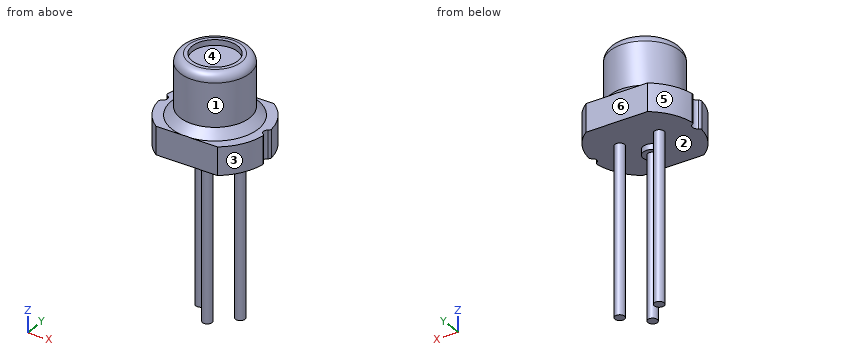
```python
from build123d import *

# Parameters (mm, degrees)
BOSS_EXTRUDE1_DEPTH = 1
SKETCH3_R           = 1.25
BOSS_EXTRUDE2_DEPTH = 2.15
CHAMFER1_SIZE       = 0.3
FILLET1_R           = 0.3
SKETCH4_R           = 0.817963918
CUT_EXTRUDE1_DEPTH  = 0.2
SKETCH5_R           = 0.175
BOSS_EXTRUDE3_DEPTH = 6
SKETCH6_R           = 0.340201154
BOSS_EXTRUDE4_DEPTH = 0.2


with BuildPart() as part:
    # Sketch1 → Boss-Extrude1 (new body)
    with BuildSketch(Plane.XY):
        with BuildLine():
            Line((-1.112834219, 1.54), (1.112834219, 1.54))
            ThreePointArc((1.112834219, 1.54), (1.63498089, 0.967903657), (1.885416667, 0.2349553))
            ThreePointArc((1.885416667, 0.2349553), (1.874554764, 0.175784903), (1.831710526, 0.133553539))
            ThreePointArc((1.831710526, 0.133553539), (1.75, 0), (1.831710526, -0.133553539))
            ThreePointArc((1.831710526, -0.133553539), (1.874554764, -0.175784903), (1.885416667, -0.2349553))
            ThreePointArc((1.885416667, -0.2349553), (1.63498089, -0.967903657), (1.112834219, -1.54))
            Line((1.112834219, -1.54), (-1.112834219, -1.54))
            ThreePointArc((-1.112834219, -1.54), (-1.626419084, -0.982222462), (-1.881, -0.268027984))
            ThreePointArc((-1.881, -0.268027984), (-1.869896042, -0.206231776), (-1.824142857, -0.163235088))
            ThreePointArc((-1.824142857, -0.163235088), (-1.72, 0), (-1.824142857, 0.163235088))
            ThreePointArc((-1.824142857, 0.163235088), (-1.869896042, 0.206231776), (-1.881, 0.268027984))
            ThreePointArc((-1.881, 0.268027984), (-1.626419084, 0.982222462), (-1.112834219, 1.54))
        make_face()
    extrude(amount=BOSS_EXTRUDE1_DEPTH)

    # Sketch3 → Boss-Extrude2 (add)
    with BuildSketch(Plane.XY.offset(1)):
        with Locations(Location((0, 0, 0), (0, 0, 180))):
            Circle(SKETCH3_R)
    extrude(amount=BOSS_EXTRUDE2_DEPTH)

    # Chamfer1
    # the kernel refuses this chamfer: 0.3 mm, written as the material it adds along each edge
    with BuildSketch(Plane(origin=(0, 0, 1), x_dir=(-1, 0, 0), z_dir=(0, 1, 0))) as chamfer1_piece_1_section:
        Polygon((1.25 + CHAMFER1_SIZE, 0), (1.25, CHAMFER1_SIZE), (1.25, 0), align=None)
    chamfer1_piece_1 = revolve(axis=Axis((0, 0, 1), (0, 0, 1)), mode=Mode.PRIVATE)
    chamfer1_piece_1 = split(chamfer1_piece_1, bisect_by=Plane(origin=(1.394706395, -1.54, 1.144706395), z_dir=(0, 1, 0)), keep=Keep.TOP, mode=Mode.PRIVATE)
    chamfer1_piece_1 = split(chamfer1_piece_1, bisect_by=Plane(origin=(1.394706395, 1.54, 1.144706395), z_dir=(0, -1, 0)), keep=Keep.TOP, mode=Mode.PRIVATE)
    add(chamfer1_piece_1)

    # Fillet1
    fillet1_edges = [part.edges().sort_by_distance(p)[0] for p in [
        (1.25, 0, 3.15),
    ]]
    fillet(fillet1_edges, radius=FILLET1_R)

    # Sketch4 → Cut-Extrude1 (cut)
    with BuildSketch(Plane.XY.offset(3.15)):
        Circle(SKETCH4_R)
    extrude(amount=-CUT_EXTRUDE1_DEPTH, mode=Mode.SUBTRACT)

    # Sketch5 → Boss-Extrude3 (add)
    with BuildSketch(Plane.XY):
        with Locations((0.715, 0.3)):
            Circle(SKETCH5_R)
        with Locations((-0.715, 0.3)):
            Circle(SKETCH5_R)
        with Locations((0, -0.415)):
            Circle(SKETCH5_R)
    extrude(amount=-BOSS_EXTRUDE3_DEPTH)

    # Sketch6 → Boss-Extrude4 (add)
    with BuildSketch(Plane(origin=(0, 0, 0), x_dir=(-1, 0, 0), z_dir=(0, 0, -1))):
        with Locations(Location((0, -0.415, 0), (0, 0, 180))):
            Circle(SKETCH6_R)
    extrude(amount=BOSS_EXTRUDE4_DEPTH)


solid = part.part
```
Check sheet for the modelled part. Datum: model origin and axes. Units: mm. Face numbers are marked on the shaded views. A direction names the side the tool comes from. Give positions to 0.01 mm unless a question says otherwise; leave off trailing zeros. Order: outer loops, then holes, each group sorted by start corner. A loop starts at its lowest first (then second) coordinate and runs counter-clockwise, first axis right, second up. Notation, with made-up numbers: M 29.5,85 L 88.5,85 A33 ccw 88.5,116 Z; hole C 54,-14 d5. An arc over 180 degrees is marked long. Answer in a Markdown table with one row per item.
1) Gauge pin test, flat ends, axial feed: P1, Ø1.4, axis at x = 1, y = -0.5, coming from the +Z side; P2, Ø1.5, axis at x = 1, z = -4, coming from the -Y side (3 decimals). Record the tip position at first contact, or that the pin passes through.
Filled sheet:
| item | result |
|---|---|
| P1 | stops at z = 3.15 |
| P2 | stops at y = 0.125 |
2) Cross-section at A-A, the plane x = 0. Enter the section's corners in (y, z).
Filled sheet:
| item | result |
|---|---|
| outline | M -1.54,0 L -0.76,0 L -0.76,-0.2 L -0.59,-0.2 L -0.59,-6 L -0.24,-6 L -0.24,-0.2 L -0.07,-0.2 L -0.07,0 L 1.54,0 L 1.54,1.01 L 1.25,1.3 L 1.25,2.85 A0.3 ccw 0.95,3.15 L 0.82,3.15 L 0.82,2.95 L -0.82,2.95 L -0.82,3.15 L -0.95,3.15 A0.3 ccw -1.25,2.85 L -1.25,1.3 L -1.54,1.01 Z |
3) Thickness scan on L1, parallel to Z at x = 0.55, y = 0.8; L2, parallel to Z at x = 1.5, y = 0.75; L3, parallel to Y at x = 0.7, z = -2. Record the ranges inside material, lowest first. Write a range as [from, to].
Filled sheet:
| item | result |
|---|---|
| L1 | z = [0, 3.15] |
| L2 | z = [0, 1] |
| L3 | y = [0.13, 0.47] |
4) Access from +Z, -Z, +X, -X, +Y, -Y to the whole of each face (thin tool, end or side, straight path). Record for the marked faces 1, 2 and 3.
Filled sheet:
| item | result |
|---|---|
| face 1 | +Z |
| face 2 | -Z |
| face 3 | +Z, -Z, +X, -Y |
5) Cross-section at B-B, the plane z = 1.75. Enter the section's corners in (x, y).
Filled sheet:
| item | result |
|---|---|
| outline | C 0,0 d2.5 |
6) Release check for a two-part mould opening along X. For the marked faces 4, 5 and 6 record: +X half, -X half, draft (parallel to the pull), parting line (faces both ways), or undercut.
Filled sheet:
| item | result |
|---|---|
| face 4 | undercut |
| face 5 | -X half |
| face 6 | draft |
7) Cross-section at C-C, the plane z = -4.5. Enter the section's corners in (x, y) (3 decimals).
Filled sheet:
| item | result |
|---|---|
| outline | C -0.715,0.3 d0.35; C 0,-0.415 d0.35; C 0.715,0.3 d0.35 |
